from build123d import *

# Parameters (mm, degrees)
SKETCH1_W                 = 20
SKETCH1_H                 = 22
BOSS_EXTRUDE1_DEPTH       = 4
M3X0_5_TAPPED_HOLE1_D     = 2.5
M3X0_5_TAPPED_HOLE1_DEPTH = 7.5
M3X0_5_TAPPED_HOLE1_TIP   = 0.751075774
M3X0_5_TAPPED_HOLE2_D     = 2.5
M3X0_5_TAPPED_HOLE2_DEPTH = 7.5
M3X0_5_TAPPED_HOLE2_TIP   = 0.751075774


with BuildPart() as part:
    # Sketch1 → Boss-Extrude1 (new body, symmetric)
    with BuildSketch(Plane(origin=(0, 0, 0), x_dir=(0, 0, -1), z_dir=(1, 0, 0))):
        Rectangle(SKETCH1_W, SKETCH1_H)
    extrude(amount=BOSS_EXTRUDE1_DEPTH, both=True)

    # M3x0.5 Tapped Hole1
    with Locations(Plane(origin=(0, 11, 0), x_dir=(1, 0, 0), z_dir=(0, 1, 0))):
        with Locations((0, 6), (0, -6)):
            Hole(M3X0_5_TAPPED_HOLE1_D / 2, depth=M3X0_5_TAPPED_HOLE1_DEPTH)
            with Locations((0, 0, -(M3X0_5_TAPPED_HOLE1_DEPTH + M3X0_5_TAPPED_HOLE1_TIP / 2))):  # 118° drill point
                Cone(0, M3X0_5_TAPPED_HOLE1_D / 2, M3X0_5_TAPPED_HOLE1_TIP, mode=Mode.SUBTRACT)

    # M3x0.5 Tapped Hole2
    with Locations(Plane(origin=(0, -11, 0), x_dir=(-1, 0, 0), z_dir=(0, -1, 0))):
        with Locations((0, -6), (0, 6)):
            Hole(M3X0_5_TAPPED_HOLE2_D / 2, depth=M3X0_5_TAPPED_HOLE2_DEPTH)
            with Locations((0, 0, -(M3X0_5_TAPPED_HOLE2_DEPTH + M3X0_5_TAPPED_HOLE2_TIP / 2))):  # 118° drill point
                Cone(0, M3X0_5_TAPPED_HOLE2_D / 2, M3X0_5_TAPPED_HOLE2_TIP, mode=Mode.SUBTRACT)


solid = part.part
Input: part model. Units: mm. Frame: model coordinates. A direction names the side the tool comes from. Give positions to 0.01 mm unless a question says otherwise; leave off trailing zeros. Write each loop counter-clockwise with the first axis right and the second up, starting at its lowest first coordinate (ties: lowest second). Pieces come first, ordered by that corner, then holes. Notation, with made-up numbers: (-4, 5.25) -> (46, 5.25) arc R31 cw to (46, 39.25) -> close; hole circle Ø6 at (68, -3). An arc over 180 degrees is marked (long way). Use one line per item in the form item = value. Start each with the question number.
1) Section query A-A on y = 7.5. Return the cut outline in (x, z), then the cut area to 3 significant figures.
2) Set-up query: faces 5 (the cylindrical face through (0.27, 7.2, 7.22)), 6 (the flat face through (0, 11, 0)), 7 (the cylindrical face through (-0.27, -7.2, -4.78)). Return all of +Z, -Z, +X, -X, +Y, -Y with unobstructed straight access to the full face (end or side cutting, diameter ignored); none if empty.
3) Pin query (flat end, axial travel): pin 1 (3 mm diameter, centred on x = 0, z = -6, fed in from -Y); pin 2 (1.5 mm diameter, centred on x = 0, z = -6, fed in from -Y); pin 3 (2 mm diameter, centred on x = 0, z = 6, fed in from +Y). Return the tip coordinate at first contact, or that it passes through.
4) Ray query, probe 1 along Z at (x, y) = (0, -8); probe 2 along X at (y, z) = (-7, 6); probe 3 along Y at (x, z) = (-0.5, 5). Return the intervals inside material, ascending. Write a range as from..to.
5) Draft query along Z for faces 1 (the flat face through (0, -11, 0)), 2 (the flat face through (0, 0, 10)), 3 (the conical face through (0.12, 2.88, 5.82)), 4 (the cylindrical face through (0.27, 7.2, -4.78)). Return one class per face: pulls with the +Z half, pulls with the -Z half, needs draft (parallel to the pull), parting line crosses it, or undercut.
Outcome:
q1.outline = (-4, -10) -> (4, -10) -> (4, 10) -> (-4, 10) -> close; hole circle Ø2.5 at (0, -6); hole circle Ø2.5 at (0, 6)
q1.area = 150 mm^2
q2.face_5 = +Y
q2.face_6 = +Z, -Z, +X, -X, +Y
q2.face_7 = -Y
q3.pin_1 = -11
q3.pin_2 = -3.2
q3.pin_3 = 3.35
q4.probe_1 = -10..-7.25, -4.75..4.75, 7.25..10
q4.probe_2 = -4..-1.25, 1.25..4
q4.probe_3 = -3.42..3.42
q5.face_1 = needs draft
q5.face_2 = pulls with the +Z half
q5.face_3 = undercut
q5.face_4 = undercut
